Here's the drawing with two shaded views (mm, measured from the low corner). I have some questions. Coordinates: 2 decimals unless noted, no trailing zeros. Write each loop counter-clockwise with the first axis right and the second up, starting at its lowest first coordinate (ties: lowest second). Pieces come first, ordered by that corner, then holes. Notation, with made-up numbers: M 89,17 L 102,17 A31 ccw 102,55 Z; hole C 5.25,-1 d1. An arc over 180 degrees is marked long. Answer as CSV lines item,"result". Start each with the question number.
Item 1: We'd pull the mould along X, two halves only. Please class the marked faces 1 and 2: +X half, -X half, draft (parallel to the pull), parting line (faces both ways), or undercut.
Item 2: I'm going to push a flat-ended pin straight in: P1, Ø5.5, axis at x = 53.848, z = 26.162, coming from the -Y side. Where does the tip first touch, or does it pass through?
Item 3: Suppose I cut it at A-A, the plane y = 2.9. Write out the boundary of the cut face in (x, z), and give its area (3 significant figures).
Item 4: If I drill on line 1 along Z through (x, y) = (54, 0.5); line 2 along Z through (x, y) = (18.5, 3.55); line 3 along Y through (x, z) = (57, 22), over which ranges is the centre line in solid material (lowest first)? Write a range as [from, to].
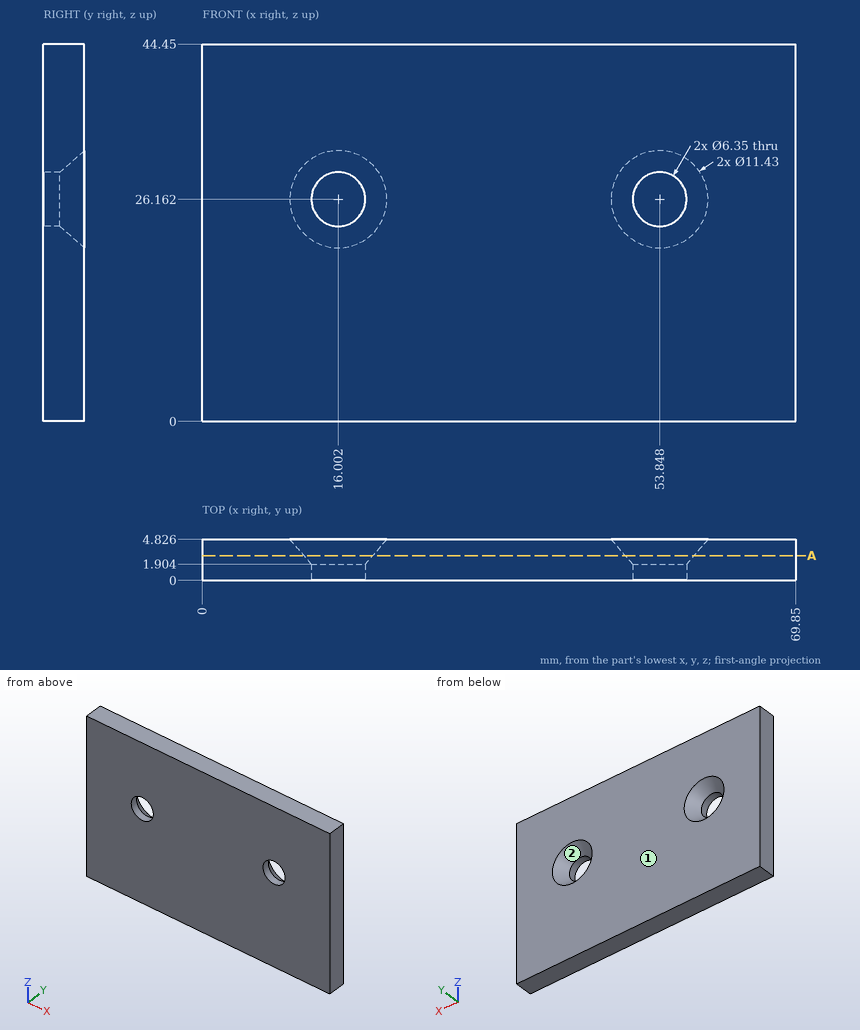
Ans:
1,face 1,"draft"
1,face 2,"undercut"
2,P1,"passes through"
3,outline,"M 0,0 L 69.85,0 L 69.85,44.45 L 0,44.45 Z; hole C 16,26.16 d8.08; hole C 53.85,26.16 d8.08"
3,area,"3,000 mm^2"
4,line 1,"z = [0, 22.99], [29.33, 44.45]"
4,line 2,"z = [0, 22.29], [30.03, 44.45]"
4,line 3,"y = [0, 4.26]"
